Check sheet for the modelled part. Datum: model origin and axes. Units: mm. A direction names the side the tool comes from. Round coordinates to 2 decimals unless told otherwise and drop trailing zeros. Order: outer loops, then holes, each group sorted by start corner. A loop starts at its lowest first (then second) coordinate and runs counter-clockwise, first axis right, second up. Notation, with made-up numbers: M 20,-13 L 71,-13 A15 ccw 71,-4 Z; hole C 29,-7.75 d9. An arc over 180 degrees is marked long. One line per item, written item: value. Start each with the question number.
(1) Cross-section at D-D, the plane x = 1.5. Enter the section's corners in (y, z), and give its area (3 significant figures).
(2) Cross-section at C-C, the plane y = 29.5. Enter the section's corners in (x, z).
(3) Access from +Z, -Z, +X, -X, +Y, -Y to the whole of each face (thin tool, end or side, straight path). Record for faces 1 (the face through (9.75, 30.71, 4.48)), 2 (the face through (0, 38, 3)), 3 (the face through (10.05, 33.92, 4.48)), 4 (the face through (-7.399, 35.688, 4.479)).
(4) Depth check by flat-ended pin: pin 1 Ø1.5 at (x, z) = (-8.5, 4.5) entering from +Y; pin 2 Ø3 at (x, z) = (-10, 2) entering from +Y; pin 3 Ø0.8 at (y, z) = (32.5, 5) entering from -X. Enter the tip coordinate at first touch or a pass-through.
(5) Thickness scan on L1, parallel to Z at x = -8, y = 36.5; L2, parallel to X at y = 32.75, z = 4.9; L3, parallel to X at y = 30.75, z = 3.1. Record the ranges inside material, lowest first.
(6) Cross-section at A-A, the plane y = 32.25. Enter the section's corners in (x, z).
from build123d import *

# Parameters (mm, degrees)
BOSS_EXTRUDE1_DEPTH = 5
BOSS_EXTRUDE2_DEPTH = 3
BOSS_EXTRUDE3_DEPTH = 1


with BuildPart() as part:
    # Sketch1 → Boss-Extrude1 (new body)
    with BuildSketch(Plane.XY):
        with BuildLine():
            Line((-5.475833864, 36.750373078), (-9.376960794, 34.595435627))
            ThreePointArc((-9.376960794, 34.595435627), (-10.056879686, 33.934547755), (-10.306619263, 33.019838718))
            Line((-10.306619263, 33.019838718), (-10.306619263, 31.999976553))
            ThreePointArc((-10.306619263, 31.999976553), (-9.779411469, 30.727184347), (-8.506619263, 30.199976553))
            Line((-8.506619263, 30.199976553), (-5.552402581, 30.199976553))
            ThreePointArc((-5.552402581, 30.199976553), (-5.398466912, 30.206570907), (-5.245659139, 30.226305653))
            ThreePointArc((-5.245659139, 30.226305653), (-2.637016879, 30.563008221), (-0.009120041, 30.674996011))
            ThreePointArc((-0.009120041, 30.674996011), (2.618776796, 30.563008221), (5.227419056, 30.226305653))
            ThreePointArc((5.227419056, 30.226305653), (5.380226829, 30.206570907), (5.534162498, 30.199976553))
            Line((5.534162498, 30.199976553), (8.493548715, 30.199976553))
            ThreePointArc((8.493548715, 30.199976553), (9.766340921, 30.727184347), (10.293548715, 31.999976553))
            Line((10.293548715, 31.999976553), (10.293548715, 33.019838718))
            ThreePointArc((10.293548715, 33.019838718), (10.043809137, 33.934547755), (9.363890246, 34.595435627))
            Line((9.363890246, 34.595435627), (5.458712815, 36.752610527))
            ThreePointArc((5.458712815, 36.752610527), (5.14978717, 36.887221852), (4.821185066, 36.961893934))
            ThreePointArc((4.821185066, 36.961893934), (-0.009071369, 37.274996263), (-4.839174836, 36.959542957))
            ThreePointArc((-4.839174836, 36.959542957), (-5.167324404, 36.884847724), (-5.475833864, 36.750373078))
        make_face()
    extrude(amount=BOSS_EXTRUDE1_DEPTH)

    # Sketch2 → Boss-Extrude2 (add)
    with BuildSketch(Plane(origin=(0, 0, 0), x_dir=(-1, 0, 0), z_dir=(0, 0, -1))):
        with BuildLine():
            ThreePointArc((10.587505912, 28.583851445), (11.993992673, 30.040837277), (12.506619263, 31.999976553))
            Line((12.506619263, 31.999976553), (12.506619263, 33.019838718))
            ThreePointArc((12.506619263, 33.019838718), (11.951642425, 35.052525467), (10.440711554, 36.521165182))
            Line((10.440711554, 36.521165182), (6.539584624, 38.676102633))
            ThreePointArc((6.539584624, 38.676102633), (5.854008048, 38.97493518), (5.124786785, 39.140924586))
            ThreePointArc((5.124786785, 39.140924586), (0.009606768, 39.474996197), (-5.105735244, 39.143414321))
            ThreePointArc((-5.105735244, 39.143414321), (-5.835962142, 38.97747636), (-6.522463575, 38.678340082))
            Line((-6.522463575, 38.678340082), (-10.427641006, 36.521165182))
            ThreePointArc((-10.427641006, 36.521165182), (-11.938571876, 35.052525467), (-12.493548715, 33.019838718))
            Line((-12.493548715, 33.019838718), (-12.493548715, 31.999976553))
            ThreePointArc((-12.493548715, 31.999976553), (-11.980256235, 30.039652429), (-10.57211338, 28.582438121))
            ThreePointArc((-10.57211338, 28.582438121), (-5.36535689, 29.998971577), (0.009611281, 30.474993977))
            ThreePointArc((0.009611281, 30.474993977), (5.382569695, 29.999329411), (10.587505912, 28.583851445))
        make_face()
        with BuildLine():
            ThreePointArc((-5.227419056, 30.226305653), (-5.380226829, 30.206570907), (-5.534162498, 30.199976553))
            Line((-5.534162498, 30.199976553), (-8.493548715, 30.199976553))
            ThreePointArc((-8.493548715, 30.199976553), (-9.766340921, 30.727184347), (-10.293548715, 31.999976553))
            Line((-10.293548715, 31.999976553), (-10.293548715, 33.019838718))
            ThreePointArc((-10.293548715, 33.019838718), (-10.043809137, 33.934547755), (-9.363890246, 34.595435627))
            Line((-9.363890246, 34.595435627), (-5.458712815, 36.752610527))
            ThreePointArc((-5.458712815, 36.752610527), (-5.14978717, 36.887221852), (-4.821185066, 36.961893934))
            ThreePointArc((-4.821185066, 36.961893934), (0.009071369, 37.274996263), (4.839174836, 36.959542957))
            ThreePointArc((4.839174836, 36.959542957), (5.167324404, 36.884847724), (5.475833864, 36.750373078))
            Line((5.475833864, 36.750373078), (9.376960794, 34.595435627))
            ThreePointArc((9.376960794, 34.595435627), (10.056879686, 33.934547755), (10.306619263, 33.019838718))
            Line((10.306619263, 33.019838718), (10.306619263, 31.999976553))
            ThreePointArc((10.306619263, 31.999976553), (9.779411469, 30.727184347), (8.506619263, 30.199976553))
            Line((8.506619263, 30.199976553), (5.552402581, 30.199976553))
            ThreePointArc((5.552402581, 30.199976553), (5.398466912, 30.206570907), (5.245659139, 30.226305653))
            ThreePointArc((5.245659139, 30.226305653), (2.637016879, 30.563008221), (0.009120041, 30.674996011))
            ThreePointArc((0.009120041, 30.674996011), (-2.618776796, 30.563008221), (-5.227419056, 30.226305653))
        make_face(mode=Mode.SUBTRACT)
    extrude(amount=-BOSS_EXTRUDE2_DEPTH)

    # Sketch6 → Boss-Extrude3 (add)
    with BuildSketch(Plane.XY.offset(5)):
        with BuildLine():
            Line((-5.475833864, 36.750373078), (-9.376960794, 34.595435627))
            ThreePointArc((-9.376960794, 34.595435627), (-10.056879686, 33.934547755), (-10.306619263, 33.019838718))
            Line((-10.306619263, 33.019838718), (-10.306619263, 31.999976553))
            ThreePointArc((-10.306619263, 31.999976553), (-9.779411469, 30.727184347), (-8.506619263, 30.199976553))
            Line((-8.506619263, 30.199976553), (-5.552402581, 30.199976553))
            ThreePointArc((-5.552402581, 30.199976553), (-5.398466912, 30.206570907), (-5.245659139, 30.226305653))
            ThreePointArc((-5.245659139, 30.226305653), (-2.637016879, 30.563008221), (-0.009120041, 30.674996011))
            ThreePointArc((-0.009120041, 30.674996011), (2.618776796, 30.563008221), (5.227419056, 30.226305653))
            ThreePointArc((5.227419056, 30.226305653), (5.380226829, 30.206570907), (5.534162498, 30.199976553))
            Line((5.534162498, 30.199976553), (8.493548715, 30.199976553))
            ThreePointArc((8.493548715, 30.199976553), (9.766340921, 30.727184347), (10.293548715, 31.999976553))
            Line((10.293548715, 31.999976553), (10.293548715, 33.019838718))
            ThreePointArc((10.293548715, 33.019838718), (10.043809137, 33.934547755), (9.363890246, 34.595435627))
            Line((9.363890246, 34.595435627), (5.458712815, 36.752610527))
            ThreePointArc((5.458712815, 36.752610527), (5.14978717, 36.887221852), (4.821185066, 36.961893934))
            ThreePointArc((4.821185066, 36.961893934), (-0.009071369, 37.274996263), (-4.839174836, 36.959542957))
            ThreePointArc((-4.839174836, 36.959542957), (-5.167324404, 36.884847724), (-5.475833864, 36.750373078))
        make_face()
    extrude(amount=BOSS_EXTRUDE3_DEPTH)


solid = part.part
Values found:
1. outline: M 30.44,0 L 39.45,0 L 39.45,3 L 37.24,3 L 37.24,6 L 30.64,6 L 30.64,3 L 30.44,3 Z
1. area: 46.8 mm^2
2. outline: M -11.63,0 L -7.67,0 L -7.67,3 L -11.63,3 Z; M 7.65,0 L 11.62,0 L 11.62,3 L 7.65,3 Z
3. face 1: +Z, +X, -Y
3. face 2: +Z
3. face 3: +Z, +X, +Y
3. face 4: +Z, -X, +Y
4. pin 1: y = 35.49
4. pin 2: y = 37.59
4. pin 3: x = -10.31
5. L1: 0 to 3
5. L2: -10.31 to 10.29
5. L3: -9.8 to 9.79
6. outline: M -12.51,0 L 12.49,0 L 12.49,3 L 10.29,3 L 10.29,6 L -10.31,6 L -10.31,3 L -12.51,3 Z
